from build123d import *

# Parameters (mm, degrees)
SKETCH1_W           = 105.7
SKETCH1_H           = 67.2
BOSS_EXTRUDE1_DEPTH = 6
SKETCH2_W           = 129.7
SKETCH2_H           = 80.2
BOSS_EXTRUDE2_DEPTH = 1.5
SKETCH3_R           = 1.5
CUT_EXTRUDE1_DEPTH  = 1.5
FILLET1_R           = 3


with BuildPart() as part:
    # Sketch1 → Boss-Extrude1 (new body)
    with BuildSketch(Plane.XY):
        Rectangle(SKETCH1_W, SKETCH1_H)
    extrude(amount=BOSS_EXTRUDE1_DEPTH)

    # Sketch2 → Boss-Extrude2 (add)
    with BuildSketch(Plane(origin=(0, 0, 0), x_dir=(-1, 0, 0), z_dir=(0, 0, -1))):
        Rectangle(SKETCH2_W, SKETCH2_H)
    extrude(amount=BOSS_EXTRUDE2_DEPTH)

    # Sketch3 → Cut-Extrude1 (cut)
    with BuildSketch(Plane.XY):
        with Locations((61.35, 36.6)):
            Circle(SKETCH3_R)
        with Locations((61.35, -36.6)):
            Circle(SKETCH3_R)
        with Locations((-61.35, -36.6)):
            Circle(SKETCH3_R)
        with Locations((-61.35, 36.6)):
            Circle(SKETCH3_R)
    extrude(amount=-CUT_EXTRUDE1_DEPTH, mode=Mode.SUBTRACT)

    # Fillet1
    fillet1_edges = [part.edges().sort_by_distance(p)[0] for p in [
        (-64.85, -40.1, -0.75),
        (-64.85, 40.1, -0.75),
        (64.85, 40.1, -0.75),
        (64.85, -40.1, -0.75),
    ]]
    fillet(fillet1_edges, radius=FILLET1_R)


solid = part.part
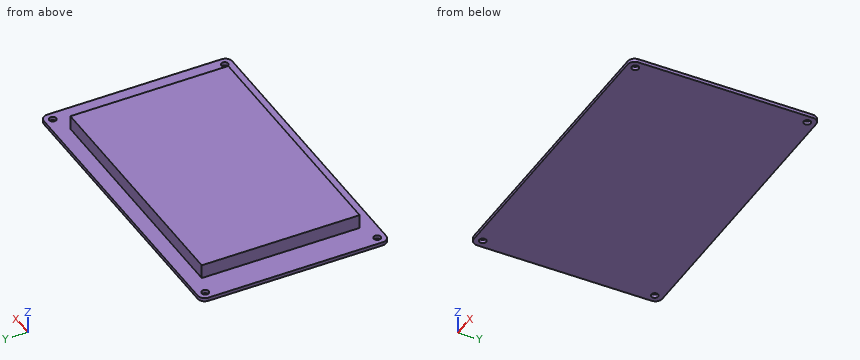
Could you check a few things on this model? Use its own coordinates, in mm. Round coordinates to 2 decimals unless told otherwise and drop trailing zeros. Order: outer loops, then holes, each group sorted by start corner. A loop starts at its lowest first (then second) coordinate and runs counter-clockwise, first axis right, second up.
(1) I'm going to push flat-ended pins straight in: pin 1 (1 mm diameter, centred on y = -25.5, z = 4.5, fed in from -X); pin 2 (3 mm diameter, centred on y = 6, z = 2.5, fed in from +X); pin 3 (1 mm diameter, centred on x = -15.5, z = 4.5, fed in from -Y). Where does each tip first touch, or does it pass through?
Response values:
pin 1: stops at x = -52.85
pin 2: stops at x = 52.85
pin 3: stops at y = -33.6
(2) Imagine slicing it at A-A (y = -14). Write out the boundary of the cut face in (x, z), plus the area to 3 significant figures.
Response values:
outline: (-64.85, -1.5) - (64.85, -1.5) - (64.85, 0) - (52.85, 0) - (52.85, 6) - (-52.85, 6) - (-52.85, 0) - (-64.85, 0) - close
area: 829 mm2
(3) Imagine slicing it at B-B (x = 27.5). Write out the boundary of the cut face in (y, z).
Response values:
outline: (-40.1, -1.5) - (40.1, -1.5) - (40.1, 0) - (33.6, 0) - (33.6, 6) - (-33.6, 6) - (-33.6, 0) - (-40.1, 0) - close
(4) Imagine slicing it at C-C (z = 2.25). Write out the boundary of the cut face in (x, y), plus the area to 3 significant figures.
Response values:
outline: (-52.85, -33.6) - (52.85, -33.6) - (52.85, 33.6) - (-52.85, 33.6) - close
area: 7,100 mm2
(5) Please list where these lines run through material, in increasing order: line 1 along Y through (x, z) = (-61.35, -0.5); line 2 along Y through (x, z) = (-18, 2); line 3 along Z through (x, y) = (25, 34).
Response values:
line 1: y = -40.1 to -38.1, -35.1 to 35.1, 38.1 to 40.1
line 2: y = -33.6 to 33.6
line 3: z = -1.5 to 0
